Here's how the part is built. I have some questions about the finished solid (model axes, mm). Face numbers are marked on the shaded views. Coordinates: 2 decimals unless noted, no trailing zeros. Write each loop counter-clockwise with the first axis right and the second up, starting at its lowest first coordinate (ties: lowest second). Pieces come first, ordered by that corner, then holes. Notation, with made-up numbers: M -13.75,83 L 8.25,83 A31 cw 8.25,114 Z; hole C 34.25,-19.5 d1. An arc over 180 degrees is marked long. Use one line per item in the form item = value. Start each with the question number.
1. I want a section at D-D, the plane y = -575. List the corners of the cut face in (x, z) for me.
2. Please list where these lines run through material, in increasing order: line 1 along Y through (x, z) = (-4, -55); line 2 along X through (y, z) = (67, -6.5); line 3 along Z through (x, y) = (-30, -123). Write a range as [from, to].
3. I'm going to push flat-ended pins straight in: pin 1 Ø2 at (x, y) = (0, -566.5) entering from -Z; pin 2 Ø18.5 at (x, y) = (-26.5, 56.5) entering from -Z; pin 3 Ø12 at (y, z) = (16, 27.5) entering from +X; pin 4 Ø8 at (x, y) = (-43.5, -634) entering from -Z. Where does each tip first touch, or does it pass through?
4. Thinking about a two-plate mould opening in Y: for the marked faces 1 and 2, which applies, released by +Y, released by -Y, zero draft, split by the parting line, or undercut?
5. I want a section at C-C, the plane z = -48.5. List the corners of the cut face in (x, y) for me.
from build123d import *

# Parameters (mm, degrees)
F0_R     = 62.61538
F1_DEPTH = 25.4
F4_DEPTH = 0.00127
F5_DEPTH = 0.127
F6_R     = 37.21538
F7_DEPTH = 975.36


with BuildPart() as f1:
    # F0 (on Front) → F1 (new body)
    with BuildSketch(Plane.XZ):
        Circle(F0_R)
    extrude(amount=F1_DEPTH)

    # F3 (on Top) → F4 (join, symmetric)
    with BuildSketch(Plane.XY):
        Polygon((61.124925, 0), (0, 173.340619), (0, 0), align=None)
        Polygon((0, 0), (0, 173.340619), (-61.587557, 0), align=None)
    extrude(amount=F4_DEPTH, both=True)

    # F2 (on Right) → F5 (join, symmetric)
    with BuildSketch(Plane.YZ):
        Polygon((0, 62.011465), (0, 0), (177.370593, 0), align=None)
        Polygon((177.370593, 0), (0, 0), (0, -62.011465), align=None)
    extrude(amount=F5_DEPTH, both=True)

    # F6 (on face) → F7 (join)
    with BuildSketch(Plane.XZ.offset(25.4)):
        Circle(F6_R)
    extrude(amount=F7_DEPTH)


solid = f1.part
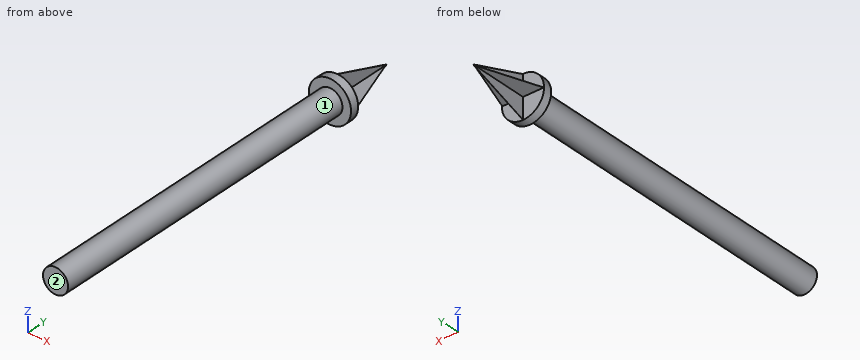
Answer list:
q1.outline = C 0,0 d74.43
q2.line_1 = [-25.4, 0]
q2.line_2 = [-0.13, 0.13]
q2.line_3 = [-22.02, 22.02]
q3.pin_1 = -37.22
q3.pin_2 = 0
q3.pin_3 = 0.13
q3.pin_4 = through
q4.face_1 = zero draft
q4.face_2 = released by -Y
q5.outline = M -39.6,-25.4 L 39.6,-25.4 L 39.6,0 L 0.13,0 L 0.13,38.65 L -0.13,38.65 L -0.13,0 L -39.6,0 Z
